Build history of the part. All positions in model axes, mm. Face numbers are marked on the shaded views. A direction names the side the tool comes from. Round coordinates to 2 decimals unless told otherwise and drop trailing zeros. Write each loop counter-clockwise with the first axis right and the second up, starting at its lowest first coordinate (ties: lowest second). Pieces come first, ordered by that corner, then holes.
1) Saw through at B-B (z = 30.48). Write the cut outline in (x, y).
2) Saw through at C-C (x = 91.44). Write the cut outline in (y, z), plus the area to 3 significant figures.
3) Saw through at D-D (x = 107). Write the cut outline in (y, z).
4) Flat gauge pins, fed straight in: pin 1 (7.5 mm diameter, centred on y = 11.5, z = 31.5, fed in from -X); pin 2 (2.5 mm diameter, centred on x = 91.44, y = 20.32, fed in from -Z); pin 3 (6.5 mm diameter, centred on x = 90.5, y = 21, fed in from -Z); pin 4 (6.5 mm diameter, centred on x = 91, y = 4, fed in from -Z). Where does each tip first touch, or does it go through?
5) Wall check: probe 1 along Y at (x, z) = (91.44, 90.65); probe 2 along Y at (x, z) = (104.5, 30.48); probe 3 along Y at (x, z) = (91, 90). Give the ranges that are in metal, low to high.
6) Which spindle directions (+Z, -Z, +X, -X, +Y, -Y) get a long thin tool onto all of the face, cutting with end or side? Do the marked faces 1 and 2. Say none if no direction does.
7) Saw through at A-A (y = 19.5). Write the cut outline in (x, z).
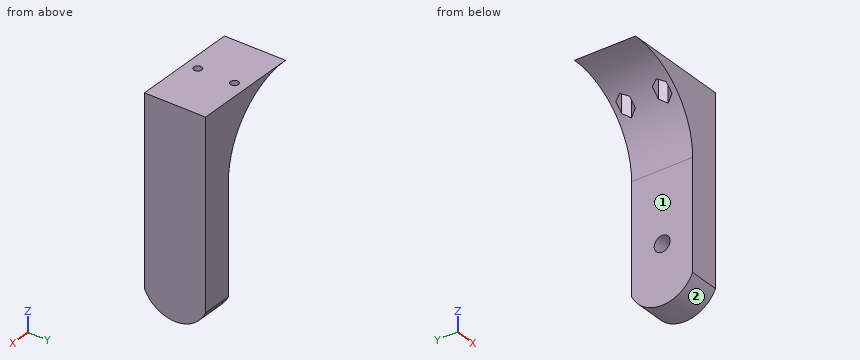
from build123d import *

# Parameters (mm, degrees)
BOSS_EXTRUDE1_DEPTH     = 25.4
SKETCH4_R               = 3.302
CUT_EXTRUDE2_DEPTH      = 7.62
SKETCH2_R               = 1.5875
SKETCH2_R_2             = 3.302
CUT_EXTRUDE3_DEPTH      = 7.62
SKETCH6_W               = 121.92
SKETCH6_H               = 12.7
BOSS_EXTRUDE2_DEPTH     = 7.62
CUT_EXTRUDE4_DEPTH      = 3.81
SKETCH10_R              = 2.921
CUT_EXTRUDE5_DEPTH      = 3.048
SKETCH11_R              = 1.5875
CUT_EXTRUDE6_DEPTH      = 96.25
CUT_EXTRUDE7_REACH      = 101.06
SKETCH12_W              = 8.89
SKETCH12_H              = 20.32
CUT_EXTRUDE8_DEPTH      = 1
CUT_EXTRUDE8_DEPTH_BACK = 122.92
CUT_EXTRUDE9_DEPTH      = 86.163777405
SKETCH16_W              = 44.941172762
SKETCH16_H              = 85.163777405
CUT_EXTRUDE10_DEPTH     = 51.8
SKETCH18_R              = 4.468004781
SKETCH18_R_2            = 4.110212911
BOSS_EXTRUDE3_DEPTH     = 2.54
SKETCH19_R              = 1.651
CUT_EXTRUDE11_DEPTH     = 2.54


with BuildPart() as part:
    # Sketch1 → Boss-Extrude1 (new body)
    with BuildSketch(Plane(origin=(0, 0, 0), x_dir=(1, 0, 0), z_dir=(0, 1, 0))):
        with BuildLine():
            Line((0, 0), (0, -59.69))
            ThreePointArc((0, -59.69), (9.299359697, -82.140640303), (31.75, -91.44))
            Line((31.75, -91.44), (69.85, -91.44))
            ThreePointArc((69.85, -91.44), (92.300640303, -82.140640303), (101.6, -59.69))
            Line((101.6, -59.69), (101.6, 0))
            Line((101.6, 0), (114.3, 0))
            Line((114.3, 0), (114.3, -99.06))
            Line((114.3, -99.06), (-7.62, -99.06))
            Line((-7.62, -99.06), (-7.62, 0))
            Line((-7.62, 0), (0, 0))
        make_face()
    extrude(amount=BOSS_EXTRUDE1_DEPTH)

    # Sketch4 → Cut-Extrude2 (cut)
    with BuildSketch(Plane.ZY.offset(-101.6)):
        with Locations((30.48, 12.7)):
            Circle(SKETCH4_R)
    extrude(amount=-CUT_EXTRUDE2_DEPTH, mode=Mode.SUBTRACT)

    # Sketch2 → Cut-Extrude3 (cut)
    with BuildSketch(Plane(origin=(0, 0, 0), x_dir=(0, 0, -1), z_dir=(1, 0, 0))):
        with Locations((-15.24, 12.7)):
            Circle(SKETCH2_R)
        with Locations((-45.72, 12.7)):
            Circle(SKETCH2_R)
        with Locations((-30.48, 12.7)):
            Circle(SKETCH2_R_2)
    extrude(amount=-CUT_EXTRUDE3_DEPTH, mode=Mode.SUBTRACT)

    # Sketch6 → Boss-Extrude2 (add)
    with BuildSketch(Plane.XY.offset(99.06)):
        with Locations((53.34, 31.75)):
            Rectangle(SKETCH6_W, SKETCH6_H)
        with Locations((53.34, -6.35)):
            Rectangle(SKETCH6_W, SKETCH6_H)
    extrude(amount=-BOSS_EXTRUDE2_DEPTH)

    # Sketch7 → Cut-Extrude4 (cut)
    with BuildSketch(Plane.XY.offset(99.06)):
        Polygon((12.284426472, 29.21), (9.901413236, 33.3375), (5.135386764, 33.3375), (2.752373528, 29.21), (5.135386764, 25.0825), (9.901413236, 25.0825), align=None)
        Polygon((103.724426472, -3.81), (101.341413236, 0.3175), (96.575386764, 0.3175), (94.192373528, -3.81), (96.575386764, -7.9375), (101.341413236, -7.9375), align=None)
    extrude(amount=-CUT_EXTRUDE4_DEPTH, mode=Mode.SUBTRACT)

    # Sketch10 → Cut-Extrude5 (cut)
    with BuildSketch(Plane.ZY.offset(7.62)):
        with Locations((15.24, 12.7)):
            Circle(SKETCH10_R)
        with Locations((45.72, 12.7)):
            Circle(SKETCH10_R)
    extrude(amount=-CUT_EXTRUDE5_DEPTH, mode=Mode.SUBTRACT)

    # Sketch11 → Cut-Extrude6 (cut, through all)
    with BuildSketch(Plane.XY.offset(95.25)):
        with Locations((7.5184, 29.21)):
            Circle(SKETCH11_R)
        with Locations((98.9584, -3.81)):
            Circle(SKETCH11_R)
    extrude(amount=-CUT_EXTRUDE6_DEPTH, mode=Mode.SUBTRACT)

    # Sketch12 → Cut-Extrude7 (cut, up to next)
    with BuildSketch(Plane.XY.offset(99.06), mode=Mode.PRIVATE) as cut_extrude7_sk1:
        with Locations((62.8396, 12.7)):
            Rectangle(SKETCH12_W, SKETCH12_H)
    cut_extrude7_tool1 = extrude(cut_extrude7_sk1.sketch, amount=-CUT_EXTRUDE7_REACH, mode=Mode.PRIVATE) & part.part
    add(cut_extrude7_tool1.solids().sort_by_distance((62.8396, 12.7, 99.06))[0], mode=Mode.SUBTRACT)

    # Sketch14 → Cut-Extrude8 (cut, two sides)
    with BuildSketch(Plane.ZY.offset(7.62)) as cut_extrude8_sk:
        with BuildLine():
            Line((14.426351463, 25.4), (0, 25.4))
            Line((0, 25.4), (0, 0))
            Line((0, 0), (14.426351463, 0))
            ThreePointArc((14.426351463, 0), (6.276222595, 12.7), (14.426351463, 25.4))
        make_face()
    extrude(amount=CUT_EXTRUDE8_DEPTH, mode=Mode.SUBTRACT)
    extrude(cut_extrude8_sk.sketch, amount=-CUT_EXTRUDE8_DEPTH_BACK, mode=Mode.SUBTRACT)

    # Sketch15 → Cut-Extrude9 (cut, through all)
    with BuildSketch(Plane(origin=(0, 0, 91.44), x_dir=(-1, 0, 0), z_dir=(0, 0, -1))):
        Polygon((-88.140443212, 20.32), (-89.790221606, 23.1775), (-93.089778394, 23.1775), (-94.739556788, 20.32), (-93.089778394, 17.4625), (-89.790221606, 17.4625), align=None)
        Polygon((-88.140443212, 5.08), (-89.790221606, 7.9375), (-93.089778394, 7.9375), (-94.739556788, 5.08), (-93.089778394, 2.2225), (-89.790221606, 2.2225), align=None)
    extrude(amount=CUT_EXTRUDE9_DEPTH, mode=Mode.SUBTRACT)

    # Sketch16 → Cut-Extrude10 (cut, through all)
    with BuildSketch(Plane(origin=(0, 38.1, 0), x_dir=(1, 0, 0), z_dir=(0, 1, 0))):
        Polygon((114.3, -99.06), (114.3, -91.44), (37.321172762, -91.44), (-7.62, -91.44), (-7.62, -99.06), align=None)
        with Locations((14.850586381, -48.858111298)):
            Rectangle(SKETCH16_W, SKETCH16_H)
    extrude(amount=-CUT_EXTRUDE10_DEPTH, mode=Mode.SUBTRACT)

    # Sketch18 → Boss-Extrude3 (add)
    with BuildSketch(Plane.XY.offset(91.44)):
        with Locations((91.226718038, 20.521889117)):
            Circle(SKETCH18_R)
        with Locations((91.757737736, 5.016113912)):
            Circle(SKETCH18_R_2)
    extrude(amount=-BOSS_EXTRUDE3_DEPTH)

    # Sketch19 → Cut-Extrude11 (cut)
    with BuildSketch(Plane.XY.offset(91.44)):
        with Locations((91.44, 20.32)):
            Circle(SKETCH19_R)
        with Locations((91.44, 5.08)):
            Circle(SKETCH19_R)
    extrude(amount=-CUT_EXTRUDE11_DEPTH, mode=Mode.SUBTRACT)


solid = part.part
Evaluation:
1. outline: (101.6, 0) - (114.3, 0) - (114.3, 25.4) - (101.6, 25.4) - (101.6, 16) - (109.22, 16) - (109.22, 9.4) - (101.6, 9.4) - close
2. outline: (0, 82.97) - (2.22, 82.97) - (2.22, 88.9) - (3.43, 88.9) - (3.43, 91.44) - (0, 91.44) - close; (6.73, 88.9) - (7.94, 88.9) - (7.94, 82.97) - (17.46, 82.97) - (17.46, 88.9) - (18.67, 88.9) - (18.67, 91.44) - (6.73, 91.44) - close; (21.97, 88.9) - (23.18, 88.9) - (23.18, 82.97) - (25.4, 82.97) - (25.4, 91.44) - (21.97, 91.44) - close
2. area: 131 mm2
3. outline: (0, 14.43) arc R13.97 ccw to (25.4, 14.43) - (25.4, 91.44) - (0, 91.44) - close; hole circle Ø6.6 at (12.7, 30.48)
4. pin 1: stops at x = 101.6
4. pin 2: passes through
4. pin 3: stops at z = 81.51
4. pin 4: stops at z = 80.01
5. probe 1: y = 0 to 3.43, 6.73 to 18.67, 21.97 to 25.4
5. probe 2: y = 0 to 9.4, 16 to 25.4
5. probe 3: y = 0 to 3.49, 6.67 to 18.73, 21.91 to 25.4
6. face 1: -Z, -X, +Y, -Y
6. face 2: -Z, +X, -X
7. outline: (69.85, 91.44) arc R31.75 cw to (88.61, 85.3) - (88.61, 88.9) - (90.01, 88.9) - (90.01, 91.44) - close; (92.87, 88.9) - (94.27, 88.9) - (94.27, 79.99) arc R31.75 cw to (101.6, 59.69) - (101.6, 8.04) - (114.3, 8.04) - (114.3, 91.44) - (92.87, 91.44) - close
